Autodesk Inventor part; units mm, degrees
ref_plane "YZ Plane" through (0, 0, 0) normal (1, 0, 0) x (0, 1, 0)
ref_plane "XZ Plane" through (0, 0, 0) normal (0, 1, 0) x (-1, 0, 0)
ref_plane "XY Plane" through (0, 0, 0) normal (0, 0, 1) x (1, 0, 0)
sketch "bASE" plane through (0, 0, 0) normal (0, 0, 1) x (1, 0, 0)
  arc A0 (-16.7865, 2.679) -> (-16.7865, -2.679) centre (-16.45, 0) ccw
  arc A1 (16.7865, -2.679) -> (16.7865, 2.679) centre (16.45, 0) ccw
  line L0 (4.4678, -4.2262) -> (16.7865, -2.679)
  line L1 (4.4678, 4.2262) -> (16.7865, 2.679)
  line L2 (-4.4678, 4.2262) -> (-16.7865, 2.679)
  line L3 (-4.4678, -4.2262) -> (-16.7865, -2.679)
  arc A2 (-4.4678, -4.2262) -> (4.4678, -4.2262) centre (0, 0) ccw
  arc A3 (4.4678, 4.2262) -> (-4.4678, 4.2262) centre (0, 0) ccw
  point P0 (0, 4.2262)
  dimension "d20" = 5.4
  dimension "d21" = 5.4
sketch "Coupling" plane through (0, 0, 0) normal (0, 0, 1) x (1, 0, 0)
  line L0 (-4.4678, 4.2262) -> (-16.7865, 2.679)
  arc A0 (4.4678, 4.2262) -> (-4.4678, 4.2262) centre (0, 0) ccw
  line L1 (4.4678, 4.2262) -> (16.7865, 2.679)
  arc A1 (16.7865, -2.679) -> (16.7865, 2.679) centre (16.45, 0) ccw
  line L2 (4.4678, -4.2262) -> (16.7865, -2.679)
  arc A2 (-4.4678, -4.2262) -> (4.4678, -4.2262) centre (0, 0) ccw
  line L3 (-4.4678, -4.2262) -> (-16.7865, -2.679)
  arc A3 (-16.7865, 2.679) -> (-16.7865, -2.679) centre (-16.45, 0) ccw
  line L4 (17.1339, 5.4452) -> (5.7046, 6.8807)
  arc A4 (5.7046, 6.8807) -> (-5.7046, 6.8807) centre (0, 0) ccw
  line L5 (-5.7046, 6.8807) -> (-17.1339, 5.4452)
  arc A5 (-17.1339, 5.4452) -> (-17.1339, -5.4452) centre (-16.45, 0) ccw
  line L6 (-17.1339, -5.4452) -> (-5.7046, -6.8807)
  arc A6 (-5.7046, -6.8807) -> (5.7046, -6.8807) centre (0, 0) ccw
  line L7 (5.7046, -6.8807) -> (17.1339, -5.4452)
  arc A7 (17.1339, -5.4452) -> (17.1339, 5.4452) centre (16.45, 0) ccw
extrude "Extrusion7" add sketch "Coupling" along normal blind 5.5 contours A0 L1 A1 L2 A2 L3 A3 L0 | A7 L7 A6 L6 A5 L5 A4 L4
extrude "Extrusion8" cut sketch "bASE" along normal blind 3
sketch "Sketch8" plane through (0, 0, 3) normal (0, 0, -1) x (-1, 0, 0)
  arc A0 (-4.4678, -4.2262) -> (4.4678, -4.2262) centre (0, 0) ccw
  circle A1 centre (0, 0) radius 4.55
  dimension "d26" = 9.1
extrude "Extrusion9" cut sketch "Sketch8" against normal blind 3
sketch "Sketch9" plane through (0, 0, 0) normal (0, 0, -1) x (-1, 0, 0)
  arc A0 (4.4678, 4.2262) -> (-4.4678, 4.2262) centre (0, 0) ccw
  line L0 (4.4678, 4.2262) -> (16.7865, 2.679)
  arc A1 (16.7865, -2.679) -> (16.7865, 2.679) centre (16.45, 0) ccw
  line L1 (16.7865, -2.679) -> (4.4678, -4.2262)
  arc A2 (-4.4678, -4.2262) -> (4.4678, -4.2262) centre (0, 0) ccw
  line L2 (-4.4678, -4.2262) -> (-16.7865, -2.679)
  arc A3 (-16.7865, 2.679) -> (-16.7865, -2.679) centre (-16.45, 0) ccw
  line L3 (-16.7865, 2.679) -> (-4.4678, 4.2262)
  line L4 (16.8276, 3.0059) -> (4.6244, 4.5387)
  arc A4 (4.6244, 4.5387) -> (-4.6244, 4.5387) centre (0, 0) ccw
  line L5 (-4.6244, 4.5387) -> (-16.8276, 3.0059)
  arc A5 (-16.8276, 3.0059) -> (-16.8276, -3.0059) centre (-16.45, 0) ccw
  line L6 (-16.8276, -3.0059) -> (-4.6244, -4.5387)
  arc A6 (-4.6244, -4.5387) -> (4.6244, -4.5387) centre (0, 0) ccw
  line L7 (4.6244, -4.5387) -> (16.8276, -3.0059)
  arc A7 (16.8276, -3.0059) -> (16.8276, 3.0059) centre (16.45, 0) ccw
extrude "Extrusion10" cut sketch "Sketch9" against normal up to surface (3 mm away)
sketch "Sketch10" plane through (0, 0, 0) normal (0, 0, -1) x (-1, 0, 0)
  arc A0 (-4.6244, -4.5387) -> (4.6244, -4.5387) centre (0, 0) ccw
  line L0 (-4.6244, -4.5387) -> (-16.8276, -3.0059)
  line L1 (-16.8276, 3.0059) -> (-4.6244, 4.5387)
  arc A1 (4.6244, 4.5387) -> (-4.6244, 4.5387) centre (0, 0) ccw
  line L2 (4.6244, 4.5387) -> (16.8276, 3.0059)
  line L3 (16.8276, -3.0059) -> (4.6244, -4.5387)
  arc A2 (-5.7046, -6.8807) -> (5.7046, -6.8807) centre (0, 0) ccw
  arc A3 (5.7046, 6.8807) -> (-5.7046, 6.8807) centre (0, 0) ccw
  arc A4 (-4.6244, -4.5387) -> (4.6244, -4.5387) centre (0, 0) ccw
  arc A5 (4.6244, 4.5387) -> (-4.6244, 4.5387) centre (0, 0) ccw
  line L4 (4.5, 7.7225) -> (4.5, 4.662)
  line L5 (4.5, -4.662) -> (4.5, -7.7225)
  line L6 (-4.5, -7.7225) -> (-4.5, -4.662)
  line L7 (-4.5, 4.662) -> (-4.5, 7.7225)
  point P0 (4.5, 0)
extrude "Extrusion11" add sketch "Sketch10" along normal blind 8
sketch "Sketch11" plane through (0, 0, 0) normal (0, 1, 0) x (-1, 0, 0)
  arc A0 (-8.5, -3.2) -> (-11.5, -3.2) centre (-10, -4) ccw
  spline S0 degree 3 poles (-11.7, -4) (-11.7, -4.2199) (-11.655, -4.4494) (-11.4803, -4.8659) (-11.3506, -5.0536) (-11.0543, -5.3499) (-10.8664, -5.4801) (-10.4488, -5.6552) (-10.2188, -5.7) (-9.7812, -5.7) (-9.5512, -5.6552) (-9.1336, -5.4801) (-8.9457, -5.3499) (-8.6494, -5.0536) (-8.5197, -4.8659) (-8.345, -4.4494) (-8.3, -4.2199) (-8.3, -3.7801) (-8.345, -3.5506) (-8.5197, -3.1341) (-8.6494, -2.9464) (-8.9457, -2.6501) (-9.1336, -2.5199) (-9.5512, -2.3448) (-9.7812, -2.3) (-10.2188, -2.3) (-10.4488, -2.3448) (-10.8664, -2.5199) (-11.0543, -2.6501) (-11.3506, -2.9464) (-11.4803, -3.1341) (-11.655, -3.5506) (-11.7, -3.7801) (-11.7, -4) knots 0 0 0 0 0.065958 0.065958 0.131917 0.131917 0.197553 0.197553 0.263189 0.263189 0.328824 0.328824 0.39446 0.39446 0.460419 0.460419 0.526377 0.526377 0.592335 0.592335 0.658294 0.658294 0.72393 0.72393 0.789566 0.789566 0.855201 0.855201 0.920837 0.920837 0.986796 0.986796 1.052754 1.052754 1.052754 1.052754
  point P0 (0, 0)
  point P1 (-11.7, -4)
extrude "Extrusion12" cut sketch "Sketch11" along normal through all both and the other way through all
fillet "Fillet1" radius 2 8 edges at (-4.5, 6.1923, 0) (-4.5, -6.1923, 0) (4.5, 6.1923, 0) (4.5, -6.1923, 0) (4.5, -6.1923, -8) (4.5, 6.1923, -8) (-4.5, 6.1923, -8) (-4.5, -6.1923, -8)
properties part number "ServoHornPocket2"
Geometry check sheet. Reference: the model listing, model coordinates, mm. A direction names the side the tool comes from. Coordinates: 2 decimals unless noted, no trailing zeros. Order: outer loops, then holes, each group sorted by start corner. A loop starts at its lowest first (then second) coordinate and runs counter-clockwise, first axis right, second up. Notation, with made-up numbers: (-25.5, -8) - (24.5, -8) arc R23 cw to (24.5, 4) - close; hole circle Ø2 at (40, 0). An arc over 180 degrees is marked (long way). One line per item, written item: value.
(1) Sectioned sample at C-C (z = -3.5). Enter the section's corners in (x, y), and give its area (3 significant figures).
Data:
outline: (-4.5, -7.72) arc R8.94 ccw to (4.5, -7.72) - (4.5, -4.66) arc R6.48 cw to (-4.5, -4.66) - close; (-4.5, 4.66) arc R6.48 cw to (4.5, 4.66) - (4.5, 7.72) arc R8.94 ccw to (-4.5, 7.72) - close
area: 47.4 mm^2
(2) Release check for a two-part mould opening along Y. For faces 6 (the face through (11.339, -6.173, 2.628)), 7 (the face through (21.937, 0.111, 2.712)), 8 (the face through (-0.07, 6.48, -2.58)) record: +Y half, -Y half, draft (parallel to the pull), parting line (faces both ways), or undercut.
Data:
face 6: -Y half
face 7: parting line
face 8: undercut
(3) Sectioned sample at D-D (x = 10.5). Enter the section's corners in (y, z).
Data:
outline: (-6.28, 0) - (-3.8, 0) - (-3.8, 3) - (3.8, 3) - (3.8, 0) - (6.28, 0) - (6.28, 5.5) - (-6.28, 5.5) - close
(4) Sectioned sample at A-A (x = 0). Enter the section's corners in (y, z), and give its area (3 significant figures).
Data:
outline: (-8.94, -8) - (-6.48, -8) - (-6.48, 3) - (-4.55, 3) - (-4.55, 5.5) - (-8.94, 5.5) - close; (4.55, 3) - (6.48, 3) - (6.48, -8) - (8.94, -8) - (8.94, 5.5) - (4.55, 5.5) - close
area: 76.0 mm^2
(5) Access from +Z, -Z, +X, -X, +Y, -Y to the whole of each face (thin tool, end or side, straight path). Record for faces 1 (the face through (0.07, -6.48, -2.58)), 2 (the face through (-11.339, 6.173, 2.628)), 3 (the face through (4.5, -6, -4)), 4 (the face through (-11.499, -6.153, 2.628)), 5 (the face through (-4.5, -6, -4)).
Data:
face 1: -Z
face 2: +Z, -Z, -X, +Y
face 3: -Z, +X, +Y, -Y
face 4: +Z, -Z, -X, -Y
face 5: -Z, -X, +Y, -Y
(6) Sectioned sample at B-B (y = 0). Enter the section's corners in (x, z), and give its area (3 significant figures).
Data:
outline: (-21.94, 0) - (-19.48, 0) - (-19.48, 3) - (-4.55, 3) - (-4.55, 5.5) - (-21.94, 5.5) - close; (4.55, 3) - (19.48, 3) - (19.48, 0) - (21.94, 0) - (21.94, 5.5) - (4.55, 5.5) - close
area: 102 mm^2
(7) Thickness scan on probe 1 along Y at (x, z) = (0, 4.15); probe 2 along Z at (x, y) = (2, 5.5); probe 3 along X at (y, z) = (0.75, 2.5). Record the ranges inside material, lowest first. Write a range as from..to.
Data:
probe 1: y = -8.94..-4.55, 4.55..8.94
probe 2: z = 3..5.5
probe 3: x = -21.89..-19.39, 19.39..21.89
(8) Depth check by flat-ended pin: pin 1 Ø1.5 at (y, z) = (-5.5, -4) entering from +X; pin 2 Ø2.5 at (y, z) = (-6.5, -3.5) entering from -X; pin 3 Ø4 at (x, y) = (13, 0.5) entering from -Z; pin 4 Ø2 at (y, z) = (-1, 1.5) entering from +X. Enter the tip coordinate at first touch or a pass-through.
Data:
pin 1: stops at x = 4.5
pin 2: stops at x = -4.5
pin 3: stops at z = 3
pin 4: stops at x = 21.94
